Read the model definition and answer for the solid it produces. Units are mm, in the model's axes. A direction names the side the tool comes from. Coordinates: 2 decimals unless noted, no trailing zeros. Loops run counter-clockwise (first coordinate to the right, second up) from the corner with the lowest first, then second, coordinate; pieces in that order, holes last.
Q1. Section D-D (x = 37.5) is taken. Give the vertices of the cut face in (y, z).
Q2. The mould has two halves that part along X. Classify faces 1 (the face through (-27, 2, -21)), 2 (the face through (57.094, 1.521, 25.219)), 3 (the face through (-1, 1, 27.5)): pulls with the +X half, pulls with the -X half, needs draft (parallel to the pull), parting line crosses it, or undercut.
Q3. Section C-C (y = 0.65) is taken. Count the separate pieces of the cut face and the enclosed holes in it, then the cut area to 3 significant figures.
Q4. Section A-A (x = -1) is taken. Give the vertices of the cut face in (y, z), then the cut area to 3 significant figures.
Q5. Straight lines are drawn through the part: line 1 (X direction, y = 1.05, z = 11.5); line 2 (X direction, y = 1.1, z = -22.5); line 3 (Z direction, x = -20, y = 1.2). For each, find the intervals that lie inside material, in ascending order.
Q6. Flat-ended cylindrical pins translate along their axes: P1, Ø1.5, axis at x = 54.5, z = 22.5, coming from the +Y side; P2, Ø0.9, axis at x = -54.5, y = 2, coming from the +Z side. Find the tip coordinate at first contact, or state that the pin passes through.
Q7. Which of the six approach directions +Z, -Z, +X, -X, +Y, -Y give full straight-line access (tool end or side, diameter ignored) to faces 4 (the face through (-1, 1, -27.5)), 5 (the face through (10, 2, -22))?
Q8. Section B-B (z = -8) is taken. Give the vertices of the cut face in (x, y), then the cut area to 3 significant figures.
from build123d import *

# Parameters (mm, degrees)
SCHIZZO1_W                   = 119
SCHIZZO1_H                   = 55
ESTRUSIONE_ESTRUSIONE1_DEPTH = 3
FORO_FILETTATO_M3X0_5_1_D    = 2.5
SCHIZZO4_W                   = 89
SCHIZZO4_H                   = 3
SCHIZZO4_W_2                 = 3
SCHIZZO4_H_2                 = 25
TAGLIO_ESTRUSIONE1_DEPTH     = 66.616308948
RACCORDO1_R                  = 8
SCHIZZO5_W                   = 34.5
SCHIZZO5_H                   = 3
TAGLIO_ESTRUSIONE2_DEPTH     = 10


with BuildPart() as part:
    # Schizzo1 → Estrusione-Estrusione1 (new body)
    with BuildSketch(Plane(origin=(0, 0, 0), x_dir=(1, 0, 0), z_dir=(0, 1, 0))):
        Rectangle(SCHIZZO1_W, SCHIZZO1_H)
    extrude(amount=ESTRUSIONE_ESTRUSIONE1_DEPTH)

    # Foro filettato M3x0.5-1 (through all)
    with Locations(Plane(origin=(0, 3, 0), x_dir=(1, 0, 0), z_dir=(0, 1, 0))):
        with Locations((-54.5, -22.5), (54.5, -22.5), (54.5, 22.5), (-54.5, 22.5)):
            Hole(FORO_FILETTATO_M3X0_5_1_D / 2)

    # Schizzo4 → Taglio-Estrusione1 (cut, through all)
    with BuildSketch(Plane(origin=(0, 3, 0), x_dir=(1, 0, 0), z_dir=(0, 1, 0))):
        with Locations((0, -22.5)):
            Rectangle(SCHIZZO4_W, SCHIZZO4_H)
        with Locations((54.5, 0)):
            Rectangle(SCHIZZO4_W_2, SCHIZZO4_H_2)
        with Locations((-54.5, 0)):
            Rectangle(SCHIZZO4_W_2, SCHIZZO4_H_2)
    extrude(amount=-TAGLIO_ESTRUSIONE1_DEPTH, mode=Mode.SUBTRACT)

    # Raccordo1
    raccordo1_edges = [part.edges().sort_by_distance(p)[0] for p in [
        (59.5, 1.5, 27.5),
        (-59.5, 1.5, 27.5),
    ]]
    fillet(raccordo1_edges, radius=RACCORDO1_R)

    # Schizzo5 → Taglio-Estrusione2 (cut)
    with BuildSketch(Plane(origin=(0, 3, 0), x_dir=(1, 0, 0), z_dir=(0, 1, 0))):
        with Locations((27.25, 22.5)):
            Rectangle(SCHIZZO5_W, SCHIZZO5_H)
        with Locations((-27.25, 22.5)):
            Rectangle(SCHIZZO5_W, SCHIZZO5_H)
    extrude(amount=-TAGLIO_ESTRUSIONE2_DEPTH, mode=Mode.SUBTRACT)


solid = part.part
Numbers:
1. outline: (0, -27.5) - (3, -27.5) - (3, -24) - (0, -24) - close; (0, -21) - (3, -21) - (3, 21) - (0, 21) - close; (0, 24) - (3, 24) - (3, 27.5) - (0, 27.5) - close
2. face 1: undercut
2. face 2: pulls with the +X half
2. face 3: needs draft
3. separate pieces: 1
3. enclosed holes: 9
3. area: 5,870 mm2
4. outline: (0, -27.5) - (3, -27.5) - (3, 21) - (0, 21) - close; (0, 24) - (3, 24) - (3, 27.5) - (0, 27.5) - close
4. area: 156 mm2
5. line 1: x = -59.5 to -56, -53 to 53, 56 to 59.5
5. line 2: x = -59.5 to -55.75, -53.25 to -44.5, -10 to 10, 44.5 to 53.25, 55.75 to 59.5
5. line 3: z = -27.5 to -24, -21 to 21, 24 to 27.5
6. P1: passes through
6. P2: stops at z = 27.08
7. face 4: -Z, +X, -X, +Y, -Y
7. face 5: +Y, -Y
8. outline: (-59.5, 0) - (-56, 0) - (-56, 3) - (-59.5, 3) - close; (-53, 0) - (53, 0) - (53, 3) - (-53, 3) - close; (56, 0) - (59.5, 0) - (59.5, 3) - (56, 3) - close
8. area: 339 mm2
